from build123d import *

# Parameters (mm, degrees)
SALIENTE_EXTRUIR1_DEPTH = 3


with BuildPart() as part:
    # Croquis1 → Saliente-Extruir1 (new body)
    with BuildSketch(Plane(origin=(0, 0, 0), x_dir=(1, 0, 0), z_dir=(0, 1, 0))):
        with BuildLine():
            Line((11, 0), (11, 7))
            Line((11, 7), (14, 7))
            Line((14, 7), (14, 0))
            Line((14, 0), (17, 0))
            Line((17, 0), (59, 0))
            Line((59, 0), (59, 20))
            Line((59, 20), (62, 20))
            Line((62, 20), (62, 0))
            Line((62, 0), (70, 0))
            ThreePointArc((70, 0), (0, 70), (-70, 0))
            Line((-70, 0), (-62, 0))
            Line((-62, 0), (-62, 20))
            Line((-62, 20), (-59, 20))
            Line((-59, 20), (-59, 0))
            Line((-59, 0), (-17, 0))
            Line((-17, 0), (-14, 0))
            Line((-14, 0), (-14, 7))
            Line((-14, 7), (-11, 7))
            Line((-11, 7), (-11, 0))
            Line((-11, 0), (-4.5, 0))
            ThreePointArc((-4.5, 0), (0, 4.5), (4.5, 0))
            Line((4.5, 0), (11, 0))
        make_face()
        Polygon((0, 11), (7, 11), (7, 14), (14.5, 14), (14.5, 31), (-14.5, 31), (-14.5, 14), (-7, 14), (-7, 11), align=None, mode=Mode.SUBTRACT)
        Polygon((24.748737342, 24.748737342), (31.819805153, 17.67766953), (33.941125497, 19.798989873), (19.798989873, 33.941125497), (17.67766953, 31.819805153), align=None, mode=Mode.SUBTRACT)
        Polygon((-24.748737342, 24.748737342), (-17.67766953, 31.819805153), (-19.798989873, 33.941125497), (-33.941125497, 19.798989873), (-31.819805153, 17.67766953), align=None, mode=Mode.SUBTRACT)
        Polygon((0, 62), (20, 62), (20, 59), (-20, 59), (-20, 62), align=None, mode=Mode.SUBTRACT)
        Polygon((55.861435714, 27.577164466), (27.577164466, 55.861435714), (29.69848481, 57.982756057), (43.840620434, 43.840620434), (57.982756057, 29.69848481), align=None, mode=Mode.SUBTRACT)
        Polygon((-27.577164466, 55.861435714), (-55.861435714, 27.577164466), (-57.982756057, 29.69848481), (-43.840620434, 43.840620434), (-29.69848481, 57.982756057), align=None, mode=Mode.SUBTRACT)
    extrude(amount=SALIENTE_EXTRUIR1_DEPTH)


solid = part.part
Build history of the part. All positions in model axes, mm. A direction names the side the tool comes from. Coordinates: 2 decimals unless noted, no trailing zeros. Write each loop counter-clockwise with the first axis right and the second up, starting at its lowest first coordinate (ties: lowest second). Pieces come first, ordered by that corner, then holes.
(1) Drill centre lines: line 1 (Z direction, x = 19, y = 2.1); line 2 (Z direction, x = 11.5, y = 2.3); line 3 (X direction, y = 2.45, z = -29). Where is each one in solid material? Low to high.
(2) Cut at C-C on x = -37. List the corners of the cut face in (y, z), and give its area (3 significant figures).
(3) Pin check, flat tips, straight feed: pin 1 Ø2 at (x, z) = (22, -57.5) entering from -Y; pin 2 Ø0.9 at (x, y) = (11, 1.5) entering from -Z; pin 3 Ø0.9 at (y, z) = (1.5, -60) entering from +X; pin 4 Ø1.5 at (y, z) = (2, -4.5) entering from +X. Stop position of each tip, or through.
(4) 3-axis set-ups, long thin cutter, end or side, ignore diameter. For faces 4 (the flat face through (60, 1, -20)), 5 (the flat face through (-41.52, 1.48, -41.92)), 6 (the flat face through (-1, 0, -35)): which of +Z, -Z, +X, -X, +Y, -Y reach the whole face in a straight line?
(5) Cut at D-D on z = -41. List the corners of the cut face in (x, y).
(6) Cut at A-A on x = 0. List the corners of the cut face in (y, z), and give its area (4 significant figures).
(7) Cut at B-B on z = -23. List the corners of the cut face in (x, y), and give its area (3 significant figures).
(8) Mould opens along Z. For faces 1 (the flat face through (-1, 3, -35)), 2 (the flat face through (12, 1, -7)), 3 (the flat face through (41.92, 1.48, -41.52)) say: pulls with the +Z half, pulls with the -Z half, needs draft (parallel to the pull), parting line crosses it, or undercut.
Working result:
1. line 1: z = -67.37 to -62, -59 to -33.14, -30.5 to 0
1. line 2: z = -69.05 to -62, -59 to -31, -14 to -7
1. line 3: x = -63.71 to -57.28, -54.44 to -24.74, -20.5 to -14.5, 14.5 to 20.5, 24.74 to 54.44, 57.28 to 63.71
2. outline: (0, -59.42) - (3, -59.42) - (3, -50.68) - (0, -50.68) - close; (0, -46.44) - (3, -46.44) - (3, 0) - (0, 0) - close
2. area: 166 mm2
3. pin 1: stops at y = 0
3. pin 2: stops at z = -69.2
3. pin 3: stops at x = 36.79
3. pin 4: stops at x = 69.9
4. face 4: +Z, +Y, -Y
4. face 5: +Y, -Y
4. face 6: +Z, -Z, +X, -X, -Y
5. outline: (-56.74, 0) - (-46.68, 0) - (-46.68, 3) - (-56.74, 3) - close; (-42.44, 0) - (42.44, 0) - (42.44, 3) - (-42.44, 3) - close; (46.68, 0) - (56.74, 0) - (56.74, 3) - (46.68, 3) - close
6. outline: (0, -70) - (3, -70) - (3, -62) - (0, -62) - close; (0, -59) - (3, -59) - (3, -31) - (0, -31) - close; (0, -11) - (3, -11) - (3, -4.5) - (0, -4.5) - close
6. area: 127.5 mm2
7. outline: (-66.11, 0) - (-30.74, 0) - (-30.74, 3) - (-66.11, 3) - close; (-26.5, 0) - (-14.5, 0) - (-14.5, 3) - (-26.5, 3) - close; (14.5, 0) - (26.5, 0) - (26.5, 3) - (14.5, 3) - close; (30.74, 0) - (66.11, 0) - (66.11, 3) - (30.74, 3) - close
7. area: 284 mm2
8. face 1: needs draft
8. face 2: pulls with the +Z half
8. face 3: undercut
